Verification items for the finished model (mm, model axes). A direction names the side the tool comes from. Round coordinates to 2 decimals unless told otherwise and drop trailing zeros. Loops run counter-clockwise (first coordinate to the right, second up) from the corner with the lowest first, then second, coordinate; pieces in that order, holes last.
from build123d import *

# Parameters (mm, degrees)
BOSS_EXTRUDE1_DEPTH = 100
FILLET2_R           = 1
FILLET3_R           = 2
SKETCH3_R           = 1.6
CUT_EXTRUDE1_DEPTH  = 214.782256883


with BuildPart() as part:
    # Sketch2 → Boss-Extrude1 (new body)
    with BuildSketch(Plane.XY):
        Polygon((182.753531726, 24.828838313), (182.753531726, -25.171161687), (170.753531726, -25.171161687), (170.753531726, -23.171161687), (180.753531726, -23.171161687), (180.753531726, 24.828838313), align=None)
    extrude(amount=BOSS_EXTRUDE1_DEPTH)

    # Fillet2
    fillet2_edges = [part.edges().sort_by_distance(p)[0] for p in [
        (170.753531726, -23.171161687, 50),
        (180.753531726, 24.828838313, 50),
    ]]
    fillet(fillet2_edges, radius=FILLET2_R)

    # Fillet3
    fillet3_edges = [part.edges().sort_by_distance(p)[0] for p in [
        (180.753531726, -23.171161687, 50),
    ]]
    fillet(fillet3_edges, radius=FILLET3_R)

    # Sketch3 → Cut-Extrude1 (cut, through all)
    with BuildSketch(Plane(origin=(0, -23.171161687, 0), x_dir=(1, 0, 0), z_dir=(0, 1, 0))):
        with Locations(Location((175.253531726, -80, 0), (0, 0, 270))):
            Circle(SKETCH3_R)
        with Locations(Location((175.253531726, -20, 0), (0, 0, 270))):
            Circle(SKETCH3_R)
    extrude(amount=-CUT_EXTRUDE1_DEPTH, mode=Mode.SUBTRACT)


solid = part.part
1. Release check for a two-part mould opening along X. For faces 1 (the face through (182.754, 0, 49)), 2 (the face through (173.692, -24.157, 19.653)), 3 (the face through (181, -4, 0)) record: released by +X, released by -X, zero draft, split by the parting line, or undercut.
2. Gauge pin test, flat ends, axial feed: P1, Ø8, axis at y = -16.5, z = 79.5, coming from the -X side; P2, Ø5, axis at y = -19.5, z = 45.5, coming from the -X side. Record the tip position at first contact, or that the pin passes through.
3. Section check A-A (z = 20). Enter the section's corners in (x, y).
4. Section check B-B (z = 54.5). Enter the section's corners in (x, y).
5. Scan lines: L1, parallel to X at y = -24.3, z = 20; L2, parallel to X at y = -14.5, z = 74.5; L3, parallel to Y at x = 175.5, z = 95. Record each from-to range of solid material in increasing order.
6. Tool access check on faces 4 (the face through (180.754, 1, 49)), 5 (the face through (173.834, -24.157, 80.738)). Record the directions out of +Z, -Z, +X, -X, +Y, -Y that give a thin tool (end or side, any length) a straight path to the whole face; none if there is none.
7. Section check C-C (y = 3). Enter the section's corners in (x, z).
Taken from the geometry:
1. face 1: released by +X
1. face 2: undercut
1. face 3: zero draft
2. P1: stops at x = 180.75
2. P2: stops at x = 180.57
3. outline: (170.75, -25.17) - (173.65, -25.17) - (173.65, -23.17) - (171.75, -23.17) arc R1 ccw to (170.75, -24.17) - close; (176.85, -25.17) - (182.75, -25.17) - (182.75, 24.83) - (181.75, 24.83) arc R1 ccw to (180.75, 23.83) - (180.75, -21.17) arc R2 cw to (178.75, -23.17) - (176.85, -23.17) - close
4. outline: (170.75, -25.17) - (182.75, -25.17) - (182.75, 24.83) - (181.75, 24.83) arc R1 ccw to (180.75, 23.83) - (180.75, -21.17) arc R2 cw to (178.75, -23.17) - (171.75, -23.17) arc R1 ccw to (170.75, -24.17) - close
5. L1: x = 170.75 to 173.65, 176.85 to 182.75
5. L2: x = 180.75 to 182.75
5. L3: y = -25.17 to -23.17
6. face 4: +Z, -Z, -X, +Y
6. face 5: +Y, -Y
7. outline: (180.75, 0) - (182.75, 0) - (182.75, 100) - (180.75, 100) - close
